from build123d import *

# Parameters (mm, degrees)
SKETCH1_R             = 29.5
SKETCH1_R_2           = 20
BOSS_EXTRUDE1_DEPTH   = 42.88
CUT_EXTRUDE1_START    = -10
SKETCH2_R             = 27.5
SKETCH2_R_2           = 20
CUT_EXTRUDE1_DEPTH    = 10
SKETCH4_W             = 40
SKETCH4_H             = 3
BOSS_EXTRUDE2_DEPTH   = 12
BOSS_EXTRUDE2_2_DEPTH = 12
CUT_EXTRUDE2_START    = -65
SKETCH5_R             = 1.6
CUT_EXTRUDE2_DEPTH    = 65
BOSS_EXTRUDE3_START   = -2
SKETCH6_W             = 130
SKETCH6_H             = 90
SKETCH6_R             = 20
SKETCH6_W_2           = 52
SKETCH6_H_2           = 59
BOSS_EXTRUDE3_DEPTH   = 2
SKETCH8_W             = 130
SKETCH8_H             = 10
BOSS_EXTRUDE4_DEPTH   = 23
BOSS_EXTRUDE5_START   = 2
SKETCH9_W             = 130
SKETCH9_H             = 90
SKETCH9_R             = 20
SKETCH9_W_2           = 52
SKETCH9_H_2           = 59
BOSS_EXTRUDE5_DEPTH   = 2
CHAMFER1_SIZE         = 3
BOSS_EXTRUDE6_DEPTH   = 130
FILLET1_R             = 2


with BuildPart() as part:
    # Sketch1 → Boss-Extrude1 (new body)
    with BuildSketch(Plane(origin=(0, 0, 0), x_dir=(1, 0, 0), z_dir=(0, 1, 0))):
        with Locations(Location((0, 0, 0), (0, 0, 270))):
            Circle(SKETCH1_R)
        with Locations(Location((0, 0, 0), (0, 0, 270))):
            Circle(SKETCH1_R_2, mode=Mode.SUBTRACT)
    extrude(amount=BOSS_EXTRUDE1_DEPTH)

    # Sketch2 → Cut-Extrude1 (cut)
    with BuildSketch(Plane(origin=(0, 42.88, 0), x_dir=(1, 0, 0), z_dir=(0, 1, 0)).offset(CUT_EXTRUDE1_START)):
        with Locations(Location((0, 0, 0), (0, 0, 270))):
            Circle(SKETCH2_R)
        with Locations(Location((0, 0, 0), (0, 0, 270))):
            Circle(SKETCH2_R_2, mode=Mode.SUBTRACT)
    extrude(amount=CUT_EXTRUDE1_DEPTH, mode=Mode.SUBTRACT)



with BuildPart() as body_2:
    # Sketch4 → Boss-Extrude2 (new body)
    with BuildSketch(Plane(origin=(0, 0, 0), x_dir=(1, 0, 0), z_dir=(0, 1, 0))):
        with Locations((60.9, 17.7)):
            Rectangle(SKETCH4_W, SKETCH4_H)
    extrude(amount=BOSS_EXTRUDE2_DEPTH)


with BuildPart() as body_3:
    # Sketch4 → Boss-Extrude2 2 (new body)
    with BuildSketch(Plane(origin=(0, 0, 0), x_dir=(1, 0, 0), z_dir=(0, 1, 0))):
        with Locations((60.9, -44.3)):
            Rectangle(SKETCH4_W, SKETCH4_H)
    extrude(amount=BOSS_EXTRUDE2_2_DEPTH)


with BuildPart() as cut_extrude2_tool:
    # Sketch5 → Cut-Extrude2 (new body)
    with BuildSketch(Plane.XY.offset(45.8).offset(CUT_EXTRUDE2_START)):
        with Locations((44.9, 4.5)):
            Circle(SKETCH5_R)
        with Locations((76.9, 4.5)):
            Circle(SKETCH5_R)
    extrude(amount=CUT_EXTRUDE2_DEPTH)


with BuildPart() as body_2_1:
    add(body_2.part)

    # Cut-Extrude2: cut by cut_extrude2_tool
    add(cut_extrude2_tool.part, mode=Mode.SUBTRACT)


with BuildPart() as body_3_1:
    add(body_3.part)

    # Cut-Extrude2: cut by cut_extrude2_tool
    add(cut_extrude2_tool.part, mode=Mode.SUBTRACT)


with BuildPart() as part_1:
    add(part.part)

    add(body_2_1.part)  # Boss-Extrude3 merges body 2

    add(body_3_1.part)  # Boss-Extrude3 merges body 3
    # Sketch6 → Boss-Extrude3 (add)
    with BuildSketch(Plane(origin=(0, 0, 0), x_dir=(1, 0, 0), z_dir=(0, 1, 0)).offset(BOSS_EXTRUDE3_START)):
        with Locations((31.9, -10.8)):
            Rectangle(SKETCH6_W, SKETCH6_H)
        with Locations(Location((0, 0, 0), (0, 0, 270))):
            Circle(SKETCH6_R, mode=Mode.SUBTRACT)
        with Locations((60.9, -13.3)):
            Rectangle(SKETCH6_W_2, SKETCH6_H_2, mode=Mode.SUBTRACT)
    extrude(amount=BOSS_EXTRUDE3_DEPTH)

    # Sketch8 → Boss-Extrude4 (add)
    with BuildSketch(Plane.XZ.offset(2)):
        with Locations((31.9, 50.8)):
            Rectangle(SKETCH8_W, SKETCH8_H)
        with Locations((31.9, -29.2)):
            Rectangle(SKETCH8_W, SKETCH8_H)
    extrude(amount=BOSS_EXTRUDE4_DEPTH)

    # Sketch9 → Boss-Extrude5 (add)
    with BuildSketch(Plane.XZ.offset(25).offset(BOSS_EXTRUDE5_START)):
        with Locations((31.9, 10.8)):
            Rectangle(SKETCH9_W, SKETCH9_H)
        with Locations(Location((0, 0, 0), (0, 0, 90))):
            Circle(SKETCH9_R, mode=Mode.SUBTRACT)
        with Locations((60.9, 13.3)):
            Rectangle(SKETCH9_W_2, SKETCH9_H_2, mode=Mode.SUBTRACT)
    extrude(amount=-BOSS_EXTRUDE5_DEPTH)

    # Chamfer1
    chamfer1_edges = [part_1.edges().sort_by_distance(p)[0] for p in [
        (40.9, 0, -17.7),
        (80.9, 0, -17.7),
        (40.9, 0, 44.3),
        (80.9, 0, 44.3),
    ]]
    chamfer(chamfer1_edges, length=CHAMFER1_SIZE)

    # Sketch11 → Boss-Extrude6 (add)
    with BuildSketch(Plane(origin=(96.9, 0, 0), x_dir=(0, 0, -1), z_dir=(1, 0, 0))):
        Polygon((34.2, -27), (34.2, -25), (56.2, -25), (56.2, 0), (59.2, 0), (59.2, -27), align=None)
    extrude(amount=-BOSS_EXTRUDE6_DEPTH)

    # Fillet1
    fillet1_edges = [part_1.edges().sort_by_distance(p)[0] for p in [
        (96.9, -12.5, -34.2),
        (-33.1, -12.5, -34.2),
        (96.9, -12.5, -56.2),
        (-33.1, -13.5, 55.8),
        (-33.1, -12.5, -56.2),
        (96.9, -13.5, 55.8),
    ]]
    fillet(fillet1_edges, radius=FILLET1_R)


solid = part_1.part
Read the model definition and answer for the solid it produces. Units are mm, in the model's axes. A direction names the side the tool comes from. Give positions to 0.01 mm unless a question says otherwise; leave off trailing zeros. Loops run counter-clockwise (first coordinate to the right, second up) from the corner with the lowest first, then second, coordinate; pieces in that order, holes last. Notation, with made-up numbers: (-22, 52.5) -> (24, 52.5) arc R13 ccw to (24, 62.5) -> close; hole circle Ø6 at (10, 17.5). An arc over 180 degrees is marked (long way). Answer as CSV lines item,"result".
Item 1: Consider line 1 (X direction, y = 4.5, z = 45.2); line 2 (Y direction, x = 76.9, z = -17.05); line 3 (Z direction, x = 87, y = -6.5). Determine where each line is inside the solid, lowest interval first. Write a range as [from, to].
Returned:
line 1,"x = [40.9, 43.3], [46.5, 75.3], [78.5, 80.9]"
line 2,"y = [-27, -25], [-2, 2.9], [6.1, 12]"
line 3,"z = [-59.2, -56.2], [-34.2, -24.2], [45.8, 55.8]"
Item 2: For faces 5 (the face through (-20.2, 32.88, 1.9)), 6 (the face through (61, 6, 45.8)), 7 (the face through (31, -13, 45.8)), 8 (the face through (61, 6, -19.2)), 9 (the face through (80.9, 7, 44)), determine the directions among +Z, -Z, +X, -X, +Y, -Y from which every point of the face is accessible in a straight line to the end or side of a thin tool.
Returned:
face 5,"+Y"
face 6,"+Z, +X, -X, +Y"
face 7,"+X, -X"
face 8,"-Z, +X, +Y"
face 9,"+Z, -Z, +X, +Y"
Item 3: Determine the mould class of faces 1 (the face through (40.9, 7, 44)), 2 (the face through (46.426, 4.981, -17.721)), 3 (the face through (33, 0, -58)), 4 (the face through (33, -27, -3)) for opening direction Y: +Y half, -Y half, draft (parallel to the pull), parting line (faces both ways), or undercut.
Returned:
face 1,"draft"
face 2,"undercut"
face 3,"+Y half"
face 4,"-Y half"
Item 4: Find section C-C on y = 4.5. Give the vertices of the cut face in (x, z), plus the area to 3 significant figures.
Returned:
outline,"circle Ø59 at (0, 0); (40.9, -19.2) -> (43.3, -19.2) -> (43.3, -16.2) -> (40.9, -16.2) -> close; (40.9, 42.8) -> (43.3, 42.8) -> (43.3, 45.8) -> (40.9, 45.8) -> close; (46.5, -19.2) -> (75.3, -19.2) -> (75.3, -16.2) -> (46.5, -16.2) -> close; (46.5, 42.8) -> (75.3, 42.8) -> (75.3, 45.8) -> (46.5, 45.8) -> close; (78.5, -19.2) -> (80.9, -19.2) -> (80.9, -16.2) -> (78.5, -16.2) -> close; (78.5, 42.8) -> (80.9, 42.8) -> (80.9, 45.8) -> (78.5, 45.8) -> close; hole circle Ø40 at (0, 0)"
area,"1,680 mm²"
Item 5: Find section B-B on z = 0. State how many separate pieces and enclosed holes the cut face has, plus the area to 3 significant figures.
Returned:
separate pieces,"6"
enclosed holes,"0"
area,"817 mm²"
Item 6: Find section A-A on y = -6.5. Give the vertices of the cut face in (x, z).
Returned:
outline,"(-33.1, -59.2) -> (96.9, -59.2) -> (96.9, -58.2) arc R2 ccw to (94.9, -56.2) -> (-31.1, -56.2) arc R2 ccw to (-33.1, -58.2) -> close; (-33.1, -32.2) arc R2 ccw to (-31.1, -34.2) -> (94.9, -34.2) arc R2 ccw to (96.9, -32.2) -> (96.9, -24.2) -> (-33.1, -24.2) -> close; (-33.1, 45.8) -> (96.9, 45.8) -> (96.9, 53.8) arc R2 ccw to (94.9, 55.8) -> (-31.1, 55.8) arc R2 ccw to (-33.1, 53.8) -> close"
Item 7: Each of these flat-tipped pins is pushed along its axis until it touches: pin 1 (6 mm diameter, centred on y = -18.5, z = -38, fed in from -X); pin 2 (6 mm diameter, centred on x = -14, y = 35, fed in from +Z); pin 3 (5 mm diameter, centred on x = 82.5, y = 7.5, fed in from -Z); pin 4 (4 mm diameter, centred on x = 44.9, y = 4.5, fed in from +Z). Where does it stop, or does it pass through?
Returned:
pin 1,"passes through"
pin 2,"stops at z = 27.37"
pin 3,"stops at z = -19.2"
pin 4,"stops at z = 45.8"
